from build123d import *

# Parameters (mm, degrees)
SKETCH_1_R            = 4
SKETCH_1_R_2          = 1.5
EXTRUDE_1_DEPTH       = 4
EXTRUDE_3_OUTLINE_R   = 4
EXTRUDE_3_OUTLINE_R_2 = 1.5
EXTRUDE_3_DEPTH       = 8
EXTRUDE_START         = 4
EXTRUDE_4_OUTLINE_R   = 6
EXTRUDE_4_OUTLINE_R_2 = 4
EXTRUDE_4_DEPTH       = 0.5
SKETCH_2_W            = 25
SKETCH_2_H            = 6
EXTRUDE_5_DEPTH       = 20
CHAMFER_1_SIZE        = 1.5
FILLET_1_R            = 2
FILLET_2_R            = 5
FILLET_4_R            = 2
SKETCH_3_R            = 1.5
CUT_EXTRUDE_1_DEPTH   = 20


# Read off the part's stored shape, not the designer's step: the extrude step, the extrude step
with BuildPart() as part:
    # Sketch 1 → Extrude 1 (new body)
    with BuildSketch(Plane.XY):
        with BuildLine():
            ThreePointArc((6, 60), (0, 66), (-6, 60))
            Line((-6, 60), (-6, -60))
            ThreePointArc((-6, -60), (0, -66), (6, -60))
            Line((6, -60), (6, 60))
        make_face()
        with Locations((0, 30)):
            Circle(SKETCH_1_R, mode=Mode.SUBTRACT)
        Circle(SKETCH_1_R, mode=Mode.SUBTRACT)
        with Locations((0, -30)):
            Circle(SKETCH_1_R, mode=Mode.SUBTRACT)
        with Locations((0, 60)):
            Circle(SKETCH_1_R_2, mode=Mode.SUBTRACT)
    extrude(amount=EXTRUDE_1_DEPTH)

    # Extrude 3 outline → Extrude 3 (add)
    # profile 1 of 4: a face of its own
    with BuildSketch(Plane.XY):
        with Locations((0, 30)):
            Circle(EXTRUDE_3_OUTLINE_R)
        with Locations((0, 30)):
            Circle(EXTRUDE_3_OUTLINE_R_2, mode=Mode.SUBTRACT)
    # profile 2 of 4: a face of its own
    with BuildSketch(Plane.XY):
        with Locations((0, 60)):
            Circle(EXTRUDE_3_OUTLINE_R)
        with Locations((0, 60)):
            Circle(EXTRUDE_3_OUTLINE_R_2, mode=Mode.SUBTRACT)
    # profile 3 of 4: a face of its own
    with BuildSketch(Plane.XY):
        Circle(EXTRUDE_3_OUTLINE_R)
        Circle(EXTRUDE_3_OUTLINE_R_2, mode=Mode.SUBTRACT)
    # profile 4 of 4: a face of its own
    with BuildSketch(Plane.XY):
        with Locations((0, -30)):
            Circle(EXTRUDE_3_OUTLINE_R)
        with Locations((0, -30)):
            Circle(EXTRUDE_3_OUTLINE_R_2, mode=Mode.SUBTRACT)
    extrude(amount=EXTRUDE_3_DEPTH)

    # Extrude 4 outline → Extrude 4 (add)
    with BuildSketch(Plane.XY.offset(EXTRUDE_START)):
        with Locations((0, 60)):
            Circle(EXTRUDE_4_OUTLINE_R)
        with Locations((0, 60)):
            Circle(EXTRUDE_4_OUTLINE_R_2, mode=Mode.SUBTRACT)
    extrude(amount=EXTRUDE_4_DEPTH)

    # Sketch 2 → Extrude 5 (add)
    with BuildSketch(Plane.XY.offset(8)):
        with Locations((0, -63)):
            Rectangle(SKETCH_2_W, SKETCH_2_H)
    extrude(amount=-EXTRUDE_5_DEPTH)

    # Chamfer 1
    chamfer_1_edges = [part.edges().sort_by_distance(p)[0] for p in [
        (6, -60, 2),
        (-6, -60, 2),
        (0, -60, 0),
        (0, -60, 4),
    ]]
    chamfer(chamfer_1_edges, length=CHAMFER_1_SIZE)

    # Fillet 1
    fillet_1_edges = [part.edges().sort_by_distance(p)[0] for p in [
        (-6, 0.75, 0),
        (0, 66, 0),
        (6, 0.75, 0),
    ]]
    fillet(fillet_1_edges, radius=FILLET_1_R)

    # Fillet 2
    fillet_2_edges = [part.edges().sort_by_distance(p)[0] for p in [
        (-12.5, -63, -12),
        (12.5, -63, -12),
    ]]
    fillet(fillet_2_edges, radius=FILLET_2_R)

    # Fillet 4
    fillet_4_edges = [part.edges().sort_by_distance(p)[0] for p in [
        (-12.5, -60, 0.5),
        (0, -60, -12),
        (12.5, -60, 0.5),
        (11.035533906, -60, -10.535533906),
        (-11.035533906, -60, -10.535533906),
    ]]
    fillet(fillet_4_edges, radius=FILLET_4_R)

    # Sketch 3 → Cut-Extrude 1 (cut)
    with BuildSketch(Plane(origin=(0, -60, 0), x_dir=(1, 0, 0), z_dir=(0, 1, 0))):
        with Locations(Location((-7.5, 7, 0), (0, 0, 270))):
            Circle(SKETCH_3_R)
        with Locations(Location((7.5, 7, 0), (0, 0, 270))):
            Circle(SKETCH_3_R)
    extrude(amount=-CUT_EXTRUDE_1_DEPTH, mode=Mode.SUBTRACT)


solid = part.part
Geometry: final body of the model. Coordinates: model frame, mm. A direction names the side the tool comes from. Give positions to 0.01 mm unless a question says otherwise; leave off trailing zeros. Order: outer loops, then holes, each group sorted by start corner. A loop starts at its lowest first (then second) coordinate and runs counter-clockwise, first axis right, second up. Notation, with made-up numbers: (-9.75, -24.75) -> (26.25, -24.75) arc R30 ccw to (26.25, 11.25) -> close; hole circle Ø7 at (-3, -30). An arc over 180 degrees is marked (long way). Put each result on its own line as item: value.
Q1. Section B-B, the plane x = 0. Count the separate pieces of the cut face and the enclosed holes in it, then the cut area to 3 significant figures.
Here are the results:
separate pieces: 5
enclosed holes: 0
area: 659 mm^2
Q2. Section C-C, the plane y = 6. Return loops of the section in (x, z).
Here are the results:
outline: (-6, 2) arc R2 ccw to (-4, 0) -> (4, 0) arc R2 ccw to (6, 2) -> (6, 4) -> (-6, 4) -> close
Q3. Pin query (flat end, axial travel): pin 1 (4 mm diameter, centred on x = 6, y = -19.5, fed in from -Z); pin 2 (2 mm diameter, centred on y = -5.5, z = 3, fed in from +X); pin 3 (2 mm diameter, centred on x = -9, z = -9, fed in from +Y). Return the tip coordinate at first contact, or that it passes through.
Here are the results:
pin 1: stops at z = 0
pin 2: stops at x = 6
pin 3: stops at y = -60
Q4. Material intervals for L1, parallel to X at y = -64.1, z = -7; L2, parallel to Z at x = 3, y = -38.5; L3, parallel to Y at x = -4.75, z = -5.5, sorted ascending.
Here are the results:
L1: x = -12.5 to -9, -6 to 6, 9 to 12.5
L2: z = 0 to 4
L3: y = -66 to -60
Q5. Section A-A, the plane y = 30. Return loops of the section in (x, z).
Here are the results:
outline: (-6, 2) arc R2 ccw to (-4, 0) -> (-1.5, 0) -> (-1.5, 8) -> (-4, 8) -> (-4, 4) -> (-6, 4) -> close; (1.5, 0) -> (4, 0) arc R2 ccw to (6, 2) -> (6, 4) -> (4, 4) -> (4, 8) -> (1.5, 8) -> close
Q6. Reachability of faces 5 (the face through (12.5, -64, 1)), 6 (the face through (-0.521, -26.034, 5.972)) from +Z, -Z, +X, -X, +Y, -Y: full face, straight path, thin tool, end or side. Return the list, or none.
Here are the results:
face 5: +Z, -Z, +X, +Y, -Y
face 6: +Z
Q7. Draft query along Z for faces 1 (the face through (2, 30, 8)), 2 (the face through (6.6, -63, -8.2)), 3 (the face through (0, 4, 0)), 4 (the face through (-0.521, 33.966, 5.972)). Return one class per face: released by +Z, released by -Z, zero draft, split by the parting line, or undercut.
Here are the results:
face 1: released by +Z
face 2: undercut
face 3: released by -Z
face 4: zero draft
